from build123d import *

# Parameters (mm, degrees)
BOSS_EXTRUDE2_DEPTH   = 58
SKETCH3_R             = 20
CUT_EXTRUDE3_DEPTH    = 105.673761331
M5X0_8_TAPPED_HOLE3_D = 4.2
M5X0_8_TAPPED_HOLE2_D = 4.2
FILLET1_R             = 4


with BuildPart() as part:
    # Sketch2 → Boss-Extrude2 (new body)
    with BuildSketch(Plane(origin=(0, 0, 0), x_dir=(1, 0, 0), z_dir=(0, 1, 0))):
        Polygon((0, 0), (0, 65), (5, 65), (5, 5), (63.030994401, 5), (63.030994401, 0), align=None)
    extrude(amount=BOSS_EXTRUDE2_DEPTH)

    # Sketch3 → Cut-Extrude3 (cut, through all)
    with BuildSketch(Plane.ZY.offset(-5)):
        with Locations((-35.5, 29)):
            Circle(SKETCH3_R)
    extrude(amount=CUT_EXTRUDE3_DEPTH, mode=Mode.SUBTRACT)

    # M5x0.8 Tapped Hole3 (through all)
    with Locations(Plane.XY):
        with Locations((11.530994401, 6.5), (11.530994401, 51.5), (56.530994401, 51.5), (56.530994401, 6.5)):
            Hole(M5X0_8_TAPPED_HOLE3_D / 2)

    # M5x0.8 Tapped Hole2 (through all)
    with Locations(Plane.ZY):
        with Locations((-11.926827682, 5.426827682), (-11.926827682, 52.573172318), (-59.073172318, 52.573172318), (-59.073172318, 5.426827682)):
            Hole(M5X0_8_TAPPED_HOLE2_D / 2)

    # Fillet1
    fillet1_edges = [part.edges().sort_by_distance(p)[0] for p in [
        (2.5, 58, -65),
        (2.5, 0, -65),
    ]]
    fillet(fillet1_edges, radius=FILLET1_R)


solid = part.part
CAD build for the part. Positions are in the model's coordinates, mm. A direction names the side the tool comes from. Round coordinates to 2 decimals unless told otherwise and drop trailing zeros. Write each loop counter-clockwise with the first axis right and the second up, starting at its lowest first coordinate (ties: lowest second). Pieces come first, ordered by that corner, then holes. Notation, with made-up numbers: M 89.25,49 L 119.25,49 A8 cw 119.25,55 Z; hole C 39.25,47 d11. An arc over 180 degrees is marked long. Put each result on its own line as item: value. Start each with the question number.
1) Saw through at A-A, the plane z = -35.5. Write the cut outline in (x, y).
2) Drill centre lines: probe 1 along Y at (x, z) = (3.7, -35.5); probe 2 along X at (y, z) = (7.5, -57); probe 3 along Z at (x, y) = (49, 10). Where is each one in solid material? Low to high. Write a range as [from, to].
3) Saw through at D-D, the plane z = -13. Write the cut outline in (x, y), and give its area (3 significant figures).
4) Saw through at C-C, the plane x = 57.5. Write the cut outline in (y, z).
5) Saw through at B-B, the plane y = 29. Write the cut outline in (x, z).
6) Pull direction Y, two halves, no side cores. Call faces 3 (the flat face through (18, 58, -4)), 4 (the cylindrical face through (54.59, 50.7, -2.53)), 5 (the flat face through (5, 29, -15)): pulls with the +Y half, pulls with the -Y half, needs draft (parallel to the pull), parting line crosses it, or undercut.
7) 3-axis set-ups, long thin cutter, end or side, ignore diameter. For faces 1 (the cylindrical face through (10.4, 8.27, -2.53)), 2 (the flat face through (34, 29, -5)): which of +Z, -Z, +X, -X, +Y, -Y reach the whole face in a straight line?
8) Pin check, flat tips, straight feed: pin 1 Ø2.5 at (y, z) = (52.57, -11.93) entering from +X; pin 2 Ø6.5 at (x, y) = (56.53, 51.5) entering from -Z. Stop position of each tip, or through.
Resolved:
1. outline: M 0,0 L 5,0 L 5,9 L 0,9 Z; M 0,49 L 5,49 L 5,58 L 0,58 Z
2. probe 1: [0, 9], [49, 58]
2. probe 2: [0, 5]
2. probe 3: [-5, 0]
3. outline: M 0,0 L 5,0 L 5,3.62 L 0,3.62 Z; M 0,7.23 L 5,7.23 L 5,50.77 L 0,50.77 Z; M 0,54.38 L 5,54.38 L 5,58 L 0,58 Z
3. area: 254 mm²
4. outline: M 0,-5 L 4.64,-5 L 4.64,0 L 0,0 Z; M 8.36,-5 L 49.64,-5 L 49.64,0 L 8.36,0 Z; M 53.36,-5 L 58,-5 L 58,0 L 53.36,0 Z
5. outline: M 0,-65 L 5,-65 L 5,-55.5 L 0,-55.5 Z; M 0,-15.5 L 5,-15.5 L 5,-5 L 63.03,-5 L 63.03,0 L 0,0 Z
6. face 3: pulls with the +Y half
6. face 4: undercut
6. face 5: needs draft
7. face 1: +Z, -Z
7. face 2: -Z, +X, +Y, -Y
8. pin 1: through
8. pin 2: z = -5
